Geometry: see drawing. Coordinates: mm, zero at the bounding-box minimum. A direction names the side the tool comes from. Round coordinates to 2 decimals unless told otherwise and drop trailing zeros. Write each loop counter-clockwise with the first axis right and the second up, starting at its lowest first coordinate (ties: lowest second). Pieces come first, ordered by that corner, then holes. Notation, with made-up numbers: M 23,34 L 51,34 A16 ccw 51,42 Z; hole C 24,-13.75 d2. An arc over 180 degrees is marked long. Use one line per item in the form item = value. Start each with the question number.
Item 1: Reachability of the marked faces 4 and 5 from +Z, -Z, +X, -X, +Y, -Y: full face, straight path, thin tool, end or side. Return the list, or none.
Item 2: Section query B-B (z = 9). Return loops of the section in (x, y).
Item 3: Pin query (flat end, axial travel): pin 1 Ø2.5 at (x, z) = (40.961, 10.234) entering from -Y; pin 2 Ø1.5 at (x, y) = (19, 5.5) entering from -Z. Return the tip coordinate at first contact, or that it passes through.
Item 4: Section query C-C (x = 16). Return loops of the section in (y, z), and give its area (3 significant figures).
Item 5: Section query D-D (y = 8). State how many separate pieces and enclosed holes the cut face has, and give its area (3 significant figures).
Item 6: Pull-direction query (Z, two-part tool) for the marked faces 1, 2 and 3; classes: pulls with the +Z half, pulls with the -Z half, needs draft (parallel to the pull), parting line crosses it, or undercut.
Item 7: Ray query, probe 1 along Z at (x, y) = (36.5, 8.25); probe 2 along X at (y, z) = (4, 72) (1 decimal); probe 3 along Z at (x, y) = (41.5, 8.25). Return the intervals inside material, ascending.
Item 8: Section query A-A (x = 23). Return loops of the section in (y, z).
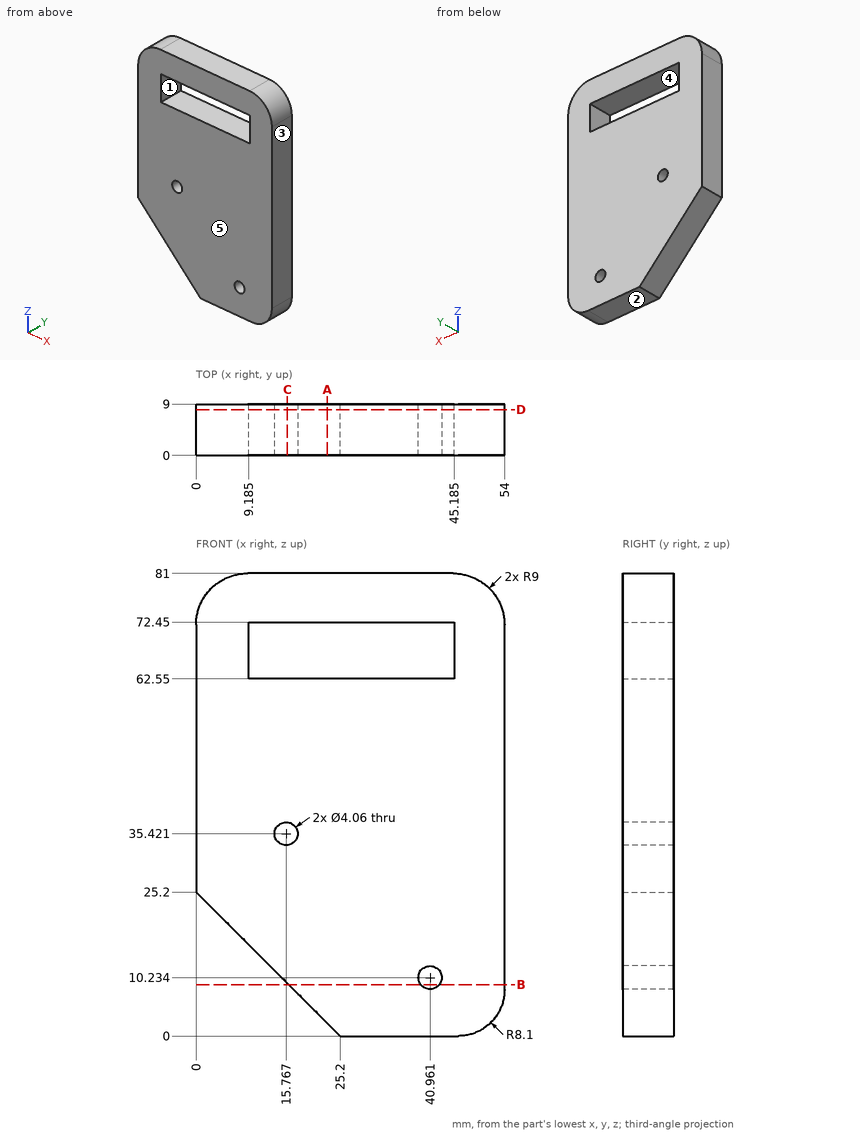
Working result:
q1.face_4 = +Y, -Y
q1.face_5 = +Z, -Z, +X, -X, -Y
q2.outline = M 16.2,0 L 39.35,0 L 39.35,9 L 16.2,9 Z; M 42.57,0 L 54,0 L 54,9 L 42.57,9 Z
q3.pin_1 = through
q3.pin_2 = 5.45
q4.outline = M 0,9.2 L 9,9.2 L 9,33.4 L 0,33.4 Z; M 0,37.44 L 9,37.44 L 9,62.55 L 0,62.55 Z; M 0,72.45 L 9,72.45 L 9,81 L 0,81 Z
q4.area = 521 mm²
q5.separate_pieces = 1
q5.enclosed_holes = 3
q5.area = 3,630 mm²
q6.face_1 = undercut
q6.face_2 = pulls with the -Z half
q6.face_3 = needs draft
q7.probe_1 = 0 to 62.55, 72.45 to 81
q7.probe_2 = 0 to 9.2, 45.2 to 54
q7.probe_3 = 0 to 8.28, 12.19 to 62.55, 72.45 to 81
q8.outline = M 0,2.2 L 9,2.2 L 9,62.55 L 0,62.55 Z; M 0,72.45 L 9,72.45 L 9,81 L 0,81 Z
